from build123d import *

# Parameters (mm, degrees)
ESQUISSE2_R             = 9
ESQUISSE2_R_2           = 5
BOSS_EXTRU_1_DEPTH      = 60
ESQUISSE3_W             = 40
ESQUISSE3_H             = 4
ESQUISSE3_W_2           = 45
ESQUISSE3_H_2           = 42
ENL_V_MAT_EXTRU_1_DEPTH = 85
CONG_1_RADIUS           = 30
CONG_1_LENGTH           = 12
ESQUISSE4_R             = 9
ESQUISSE4_R_2           = 8.001463265
ENL_V_MAT_EXTRU_2_DEPTH = 85
ESQUISSE5_R             = 13
ENL_V_MAT_EXTRU_3_DEPTH = 12


with BuildPart() as part:
    # Esquisse2 → Boss.-Extru.1 (new body)
    with BuildSketch(Plane(origin=(0, 0, 0), x_dir=(0, 0, -1), z_dir=(1, 0, 0))):
        with BuildLine():
            Line((0, -25.5), (-50, -25.5))
            Line((-50, -25.5), (-50, -12.5))
            Line((-50, -12.5), (-62, -12.5))
            Line((-62, -12.5), (-62, 17.5))
            ThreePointArc((-62, 17.5), (-92, 34.820508076), (-92, 0.179491924))
            Line((-92, 0.179491924), (-92, -31.5))
            Line((-92, -31.5), (-100, -31.5))
            Line((-100, -31.5), (-100, -37.5))
            Line((-100, -37.5), (0, -37.5))
            Line((0, -37.5), (0, -25.5))
        make_face()
        with Locations((-82, 17.5)):
            Circle(ESQUISSE2_R, mode=Mode.SUBTRACT)
        with Locations((-77, -25.5)):
            Circle(ESQUISSE2_R_2, mode=Mode.SUBTRACT)
    extrude(amount=BOSS_EXTRU_1_DEPTH)

    # Esquisse3 → Enlèv. mat.-Extru.1 (cut, symmetric)
    with BuildSketch(Plane(origin=(0, 0, 62), x_dir=(-1, 0, 0), z_dir=(0, 0, -1))):
        with Locations((-30, -35.5)):
            Rectangle(ESQUISSE3_W, ESQUISSE3_H)
        with Locations((-30, 16.5)):
            Rectangle(ESQUISSE3_W_2, ESQUISSE3_H_2)
    extrude(amount=ENL_V_MAT_EXTRU_1_DEPTH, both=True, mode=Mode.SUBTRACT)

    # Congé1: full round fillet: the end face becomes a half cylinder, R = half its width
    cong_1_face = Plane((30, -31.5, 0), x_dir=(0, -1, 0), z_dir=(0, 0, -1))  # on the end face: x along it, z out of the body
    cong_1_slab = cong_1_face.offset(-CONG_1_RADIUS / 2) * Box(CONG_1_LENGTH, 2 * CONG_1_RADIUS, CONG_1_RADIUS, mode=Mode.PRIVATE)  # the body's end, R deep
    cong_1_round = Plane((30, -31.5, 30), x_dir=(0, 0, -1), z_dir=(0, -1, 0)) * Cylinder(CONG_1_RADIUS, CONG_1_LENGTH, mode=Mode.PRIVATE)  # its axis R under the face
    add(cong_1_slab - cong_1_round, mode=Mode.SUBTRACT)

    # Esquisse4 → Enlèv. mat.-Extru.2 (cut, symmetric)
    with BuildSketch(Plane(origin=(0, -4.5, 0), x_dir=(1, 0, 0), z_dir=(0, 1, 0))):
        with Locations(Location((30, -78, 0), (0, 0, 270))):
            Circle(ESQUISSE4_R)
        with Locations(Location((30, -30, 0), (0, 0, 270))):
            Circle(ESQUISSE4_R_2)
    extrude(amount=ENL_V_MAT_EXTRU_2_DEPTH, both=True, mode=Mode.SUBTRACT)

    # Esquisse5 → Enlèv. mat.-Extru.3 (cut)
    with BuildSketch(Plane(origin=(0, 0, 50), x_dir=(-1, 0, 0), z_dir=(0, 0, -1))):
        with Locations((-30, -12.5)):
            Circle(ESQUISSE5_R)
    extrude(amount=-ENL_V_MAT_EXTRU_3_DEPTH, mode=Mode.SUBTRACT)


solid = part.part
Verification items for the finished model (mm, model axes). A direction names the side the tool comes from. Coordinates: 2 decimals unless noted, no trailing zeros. Write each loop counter-clockwise with the first axis right and the second up, starting at its lowest first coordinate (ties: lowest second). Pieces come first, ordered by that corner, then holes. Notation, with made-up numbers: (85.5, 85) - (138.5, 85) arc R22 cw to (138.5, 109) - close; hole circle Ø2 at (69, 30). An arc over 180 degrees is marked (long way). Answer as a JSON object with one key per item and string values.
(1) Thickness scan on line 1 along Z through (x, y) = (57.75, 17.5); line 2 along Y through (x, z) = (15, 77); line 3 along X through (y, z) = (-19, 78). Record the ranges inside material, lowest first.
Report:
{"line 1": "62 to 73, 91 to 102", "line 2": "-33.5 to -30.5, -20.5 to -4.5", "line 3": "0 to 21, 39 to 60"}
(2) Gauge pin test, flat ends, axial feed: pin 1 Ø4.5 at (y, z) = (-36.5, 71) entering from -X; pin 2 Ø20 at (x, z) = (31.5, 36) entering from -Y; pin 3 Ø2 at (x, y) = (6.5, 27) entering from -Z; pin 4 Ø4 at (x, y) = (38.5, -20.5) entering from -Z. Record the tip position at first contact, or that the pin passes through.
Report:
{"pin 1": "x = 0", "pin 2": "y = -33.5", "pin 3": "z = 63.9", "pin 4": "z = 50"}
(3) Cross-section at A-A on z = 76.5. Give the number of separate pieces and of enclosed holes in the cut face, plus the area to 3 significant figures.
Report:
{"separate pieces": "6", "enclosed holes": "0", "area": "1,290 mm^2"}
(4) Cross-section at D-D on z = 40. Record the cut outline in (x, y), plus the area to 3 significant figures.
Report:
{"outline": "(0, -37.5) - (10, -37.5) - (10, -33.5) - (50, -33.5) - (50, -37.5) - (60, -37.5) - (60, -25.5) - (0, -25.5) - close", "area": "560 mm^2"}
(5) Cross-section at C-C on y = 30.5. Record the cut outline in (x, z).
Report:
{"outline": "(0, 66.8) - (7.5, 66.8) - (7.5, 97.2) - (0, 97.2) - close; (52.5, 66.8) - (60, 66.8) - (60, 97.2) - (52.5, 97.2) - close"}
(6) Cross-section at B-B on y = -9.5. Record the cut outline in (x, z).
Report:
{"outline": "(0, 62) - (60, 62) - (60, 92) - (0, 92) - close; hole circle Ø18 at (30, 78)"}
(7) Tool access check on faces 1 (the flat face through (48, -19, 50)), 2 (the flat face through (52.5, 16.2, 72.8)), 3 (the flat face through (10, -36, 54)), 4 (the flat face through (30, -33, 100)). Record the directions out of +Z, -Z, +X, -X, +Y, -Y that give a thin tool (end or side, any length) a straight path to the whole face; none if there is none.
Report:
{"face 1": "-Z, +X, -X, +Y", "face 2": "+Z, -Z, +Y", "face 3": "+Z, -Z, -Y", "face 4": "+Z, +X, -X, -Y"}
(8) Mould release check, pull along Y, two halves, no side actions. Record for faces 5 (the flat face through (8, -12.5, 56)), 6 (the flat face through (30, -7, 62)), 7 (the flat face through (30, -31.5, 96)), 8 (the flat face through (5, -37.5, 54)): pulls with the +Y half, pulls with the -Y half, needs draft (parallel to the pull), parting line crosses it, or undercut.
Report:
{"face 5": "pulls with the +Y half", "face 6": "needs draft", "face 7": "undercut", "face 8": "pulls with the -Y half"}
